Verification items for the finished model (mm, model axes). Coordinates: 2 decimals unless noted, no trailing zeros. Order: outer loops, then holes, each group sorted by start corner. A loop starts at its lowest first (then second) coordinate and runs counter-clockwise, first axis right, second up. Notation, with made-up numbers: M 55,59.5 L 90,59.5 A33 ccw 90,95.5 Z; hole C 67.5,49 d10. An arc over 180 degrees is marked long. Return JSON: item names as keys, results as strings.
```python
from build123d import *

# Parameters (mm, degrees)
F1_DEPTH       = 52.5
F2_W           = 21.210102
F2_H           = 4.993801
F3_DEPTH       = 5
F5_D           = 5
F5_DEPTH       = 6.1
F5_CBORE_D     = 8.1
F5_CBORE_DEPTH = 3.2
F6_D           = 5
F6_DEPTH       = 6.1
F6_CBORE_D     = 8.1
F6_CBORE_DEPTH = 3.2


with BuildPart() as f1:
    # F0 (on Front) → F1 (new body, symmetric)
    with BuildSketch(Plane.XZ):
        Polygon((-7.799124, -1.9758), (-7.799124, -3.012683), (7.814229, -3.012683), (7.814229, -1.9758), (10.609305, 0.789221), (8.38992, 3.032728), (-8.401712, 3.032728), (-10.609227, 0.789221), align=None)
    extrude(amount=F1_DEPTH, both=True)

    # F2 (on Top) → F3 (cut)
    with BuildSketch(Plane.XY):
        with Locations((0.005642, -4.996805)):
            Rectangle(F2_W, F2_H)
        with Locations((0.005642, -14.996806)):
            Rectangle(F2_W, F2_H)
        with Locations((0.005642, -24.996806)):
            Rectangle(F2_W, F2_H)
        with Locations((0.005642, -34.996805)):
            Rectangle(F2_W, F2_H)
        with Locations((0.005642, -44.996805)):
            Rectangle(F2_W, F2_H)
        with Locations((0.005642, 5.003195)):
            Rectangle(F2_W, F2_H)
        with Locations((0.005642, 15.003194)):
            Rectangle(F2_W, F2_H)
        with Locations((0.005642, 25.003194)):
            Rectangle(F2_W, F2_H)
        with Locations((0.005642, 35.003194)):
            Rectangle(F2_W, F2_H)
        with Locations((0.005642, 45.003194)):
            Rectangle(F2_W, F2_H)
    extrude(amount=F3_DEPTH, mode=Mode.SUBTRACT)

    # F5
    with Locations(Plane.XY.offset(3.032728)):
        with Locations((0, 42.994596)):
            CounterBoreHole(F5_D / 2, F5_CBORE_D / 2, F5_CBORE_DEPTH, depth=F5_DEPTH)

    # F6
    with Locations(Plane.XY.offset(3.032728)):
        with Locations((0, -42.977002)):
            CounterBoreHole(F6_D / 2, F6_CBORE_D / 2, F6_CBORE_DEPTH, depth=F6_DEPTH)


solid = f1.part
```
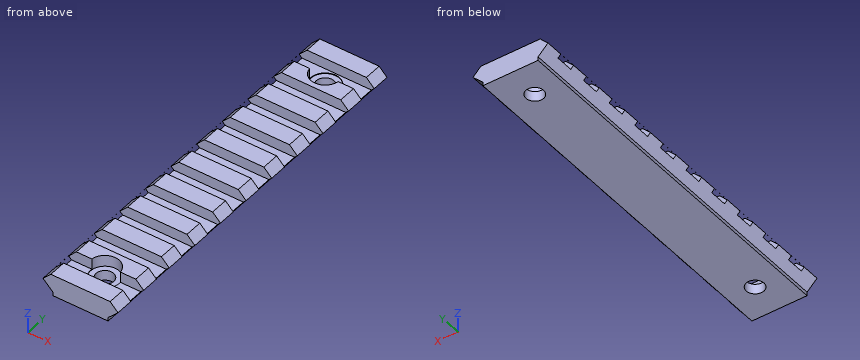
Q1. Go/stop test with flat-tipped pins: pin 1 (4 mm diameter, centred on x = -1, y = 5, fed in from +Z); pin 2 (2.5 mm diameter, centred on x = 2, y = 44, fed in from +Z). Record where each tip stops, or that it passes through.
Values:
{"pin 1": "z = 0", "pin 2": "z = -0.17"}
Q2. Cross-section at A-A, the plane x = 0. State how many separate pieces and enclosed holes the cut face has, and give its area (3 significant figures).
Values:
{"separate pieces": "3", "enclosed holes": "0", "area": "431 mm^2"}
Q3. Cross-section at B-B, the plane y = 19. Record the boundary of the cut face in (x, z).
Values:
{"outline": "M -10.61,0.79 L -7.8,-1.98 L -7.8,-3.01 L 7.81,-3.01 L 7.81,-1.98 L 10.61,0.79 L 8.39,3.03 L -8.4,3.03 Z"}
Q4. Material ranges on line 1 along Y through (x, z) = (0, -2.1); line 2 along X through (y, z) = (-46, -2.25); line 3 along Z through (x, y) = (3.5, -45.5), recorded low to high.
Values:
{"line 1": "-52.5 to -45.48, -40.48 to 40.49, 45.49 to 52.5", "line 2": "-7.8 to 7.81", "line 3": "-3.01 to 0"}
